```python
from build123d import *

# Parameters (mm, degrees)
SKETCH1_R           = 26.5
BOSS_EXTRUDE1_DEPTH = 34
FILLET1_R           = 3
CUT_EXTRUDE1_REACH  = 36
SKETCH2_R           = 3.5


with BuildPart() as part:
    # Sketch1 → Boss-Extrude1 (new body)
    with BuildSketch(Plane.XY):
        Circle(SKETCH1_R)
    extrude(amount=BOSS_EXTRUDE1_DEPTH)

    # Fillet1
    fillet1_edges = [part.edges().sort_by_distance(p)[0] for p in [
        (-26.5, 0, 0),
        (-26.5, 0, 34),
    ]]
    fillet(fillet1_edges, radius=FILLET1_R)

    # Sketch2 → Cut-Extrude1 (cut, up to next)
    with BuildSketch(Plane.XY.offset(34), mode=Mode.PRIVATE) as cut_extrude1_sk1:
        Circle(SKETCH2_R)
    cut_extrude1_tool1 = extrude(cut_extrude1_sk1.sketch, amount=-CUT_EXTRUDE1_REACH, mode=Mode.PRIVATE) & part.part
    add(cut_extrude1_tool1.solids().sort_by_distance((0, 0, 34))[0], mode=Mode.SUBTRACT)


solid = part.part
```
The model under review builds one solid part; all positions refer to its coordinate system, in mm. Round coordinates to 2 decimals unless told otherwise and drop trailing zeros. Loops run counter-clockwise (first coordinate to the right, second up) from the corner with the lowest first, then second, coordinate; pieces in that order, holes last.
Item 1: Take a section at A-A (y = 0). Write out the cut boundary in (x, z), then the cut area to 3 significant figures.
Determined:
outline: (-26.5, 3) arc R3 ccw to (-23.5, 0) - (-3.5, 0) - (-3.5, 34) - (-23.5, 34) arc R3 ccw to (-26.5, 31) - close; (3.5, 0) - (23.5, 0) arc R3 ccw to (26.5, 3) - (26.5, 31) arc R3 ccw to (23.5, 34) - (3.5, 34) - close
area: 1,560 mm2
Item 2: For line 1 (Y direction, x = 0, z = 26); line 2 (Y direction, x = -3, z = 4); line 3 (Y direction, x = -5, z = 24.5), list the stretches that pass through material, from the lowest coordinate up.
Determined:
line 1: y = -26.5 to -3.5, 3.5 to 26.5
line 2: y = -26.33 to -1.8, 1.8 to 26.33
line 3: y = -26.02 to 26.02
Item 3: Mouldability with a two-part tool opening along Y and no side actions: class faces 1 (the face through (0, -5, 34)), 2 (the face through (14.246, 22.345, 16.804)), 3 (the face through (3.233, -1.341, 17.238)) as released by +Y, released by -Y, zero draft, split by the parting line, or undercut.
Determined:
face 1: zero draft
face 2: split by the parting line
face 3: undercut
Item 4: Take a section at C-C (z = 22.5). Write out the cut boundary in (x, y).
Determined:
outline: circle Ø53 at (0, 0); hole circle Ø7 at (0, 0)
Item 5: Clearance check with flat-ended pins moving along their axes: pin 1 Ø8 at (x, z) = (20, 19) entering from -Y; pin 2 Ø8 at (y, z) = (-6.5, 10) entering from -X; pin 3 Ø12 at (y, z) = (-11.5, 28) entering from -X. State where each tip first meets the part, or that it passes through.
Determined:
pin 1: stops at y = -21.12
pin 2: stops at x = -26.38
pin 3: stops at x = -25.92
